Work out the finished part from the listing and answer in its coordinate system (mm). Coordinates: 2 decimals unless noted, no trailing zeros. Write each loop counter-clockwise with the first axis right and the second up, starting at its lowest first coordinate (ties: lowest second). Pieces come first, ordered by that corner, then holes. Notation, with made-up numbers: (54, 61) - (70, 61) arc R9 cw to (70, 77) - close; hole circle Ø3 at (25.5, 28). An arc over 180 degrees is marked (long way). Use a Markdown table: item, result. Add a question column.
(1) Find the intervals of material crossed by line 1 (X direction, y = 2.7, z = -50); line 2 (Z direction, x = 26, y = 1); line 3 (Z direction, x = 54.5, y = 2.7), in increasing order. Write a range as from..to.
(2) The part is cut by section C-C, the plane y = 3.65. Give the vertices of the cut face in (x, z), then the cut area to 3 significant figures.
(3) For a pull along Z with two mould halves and no side action, classify faces 1 (the face through (26.42, 2.46, -57.94)), 2 (the face through (8.24, 2.46, -51.44)), 3 (the face through (32, 0, -28)) as released by +Z, released by -Z, zero draft, split by the parting line, or undercut.
(4) The part is cut by section D-D, the plane x = 14. Give the vertices of the cut face in (y, z), then the cut area to 3 significant figures.
(5) The part is cut by section B-B, the plane z = -55. Give the vertices of the cut face in (x, y).
(6) The part is cut by section A-A, the plane x = 32.5. Give the vertices of the cut face in (y, z).
(7) Given pin 1 Ø1 at (y, z) = (2, -45.5) entering from -X, flat-ended and moving along its own axis, determine where the tip first touches the part or whether it passes through.
from build123d import *

# Parameters (mm, degrees)
SKETCH1_R           = 10
BOSS_EXTRUDE1_DEPTH = 5


with BuildPart() as part:
    # Sketch1 → Boss-Extrude1 (new body)
    with BuildSketch(Plane(origin=(0, 0, 0), x_dir=(1, 0, 0), z_dir=(0, 1, 0))):
        with BuildLine():
            Line((0, 35), (0, 0))
            Line((0, 0), (65, 0))
            Line((65, 0), (65, 35))
            Line((65, 35), (48.959951679, 67.319800692))
            ThreePointArc((48.959951679, 67.319800692), (32.618975384, 71.269620496), (16.252437814, 67.427091283))
            Line((16.252437814, 67.427091283), (0, 35))
        make_face()
        with Locations(Location((32.5, 50, 0), (0, 0, 270))):
            Circle(SKETCH1_R, mode=Mode.SUBTRACT)
    extrude(amount=BOSS_EXTRUDE1_DEPTH)


solid = part.part
Model answer:
| question | item | result |
|---|---|---|
| 1 | line 1 | 7.52..22.5, 42.5..57.56 |
| 1 | line 2 | -70.68..-57.6, -42.4..0 |
| 1 | line 3 | -56.16..0 |
| 2 | outline | (0, -35) - (16.25, -67.43) arc R36.27 ccw to (48.96, -67.32) - (65, -35) - (65, 0) - (0, 0) - close; hole circle Ø20 at (32.5, -50) |
| 2 | area | 3,630 mm^2 |
| 3 | face 1 | undercut |
| 3 | face 2 | released by -Z |
| 3 | face 3 | zero draft |
| 4 | outline | (0, -62.93) - (5, -62.93) - (5, 0) - (0, 0) - close |
| 4 | area | 315 mm^2 |
| 5 | outline | (10.02, 0) - (23.84, 0) - (23.84, 5) - (10.02, 5) - close; (41.16, 0) - (55.07, 0) - (55.07, 5) - (41.16, 5) - close |
| 6 | outline | (0, -71.27) - (5, -71.27) - (5, -60) - (0, -60) - close; (0, -40) - (5, -40) - (5, 0) - (0, 0) - close |
| 7 | pin 1 | x = 5.01 |
